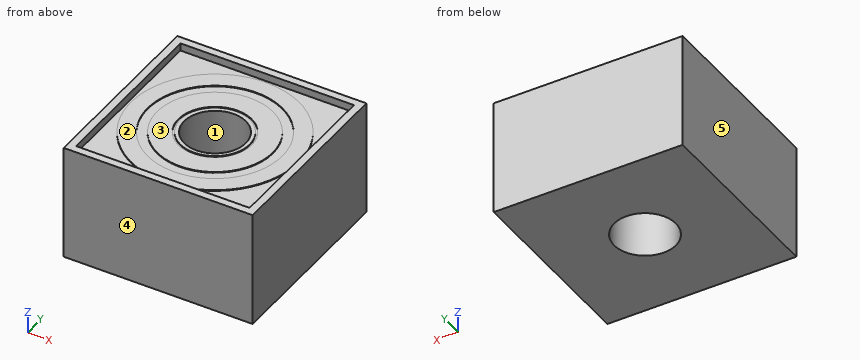
```python
from build123d import *

# Parameters (mm, degrees)
SKETCH2_W                = 24.5
SKETCH2_H                = 24.5
SKETCH2_W_2              = 22.5
SKETCH2_H_2              = 22.5
BOSS_EXTRUDE1_DEPTH      = 15
SKETCH3_W                = 22.5
SKETCH3_H                = 22.5
BOSS_EXTRUDE2_DEPTH      = 14
BOSS_EXTRUDE4_DEPTH      = 0.1
BOSS_EXTRUDE4_DEPTH_BACK = 6.9
SKETCH4_R                = 10.9
SKETCH4_R_2              = 8.730342775
SKETCH4_R_3              = 7.5
SKETCH4_R_4              = 4.75
SKETCH4_R_5              = 4.5
SKETCH4_R_6              = 4
CUT_EXTRUDE1_START       = -15
SKETCH6_R                = 4
CUT_EXTRUDE1_DEPTH       = 15


with BuildPart() as part:
    # Sketch2 → Boss-Extrude1 (new body)
    with BuildSketch(Plane.XY):
        Rectangle(SKETCH2_W, SKETCH2_H)
        Rectangle(SKETCH2_W_2, SKETCH2_H_2, mode=Mode.SUBTRACT)
    extrude(amount=BOSS_EXTRUDE1_DEPTH)

    # Sketch3 → Boss-Extrude2 (add)
    with BuildSketch(Plane.XY):
        Rectangle(SKETCH3_W, SKETCH3_H)
    extrude(amount=BOSS_EXTRUDE2_DEPTH)

    # Sketch4 → Boss-Extrude4 (add, two sides: drawn at the far end of the back side and taken through both)
    # profile 1 of 3: a face of its own
    with BuildSketch(Plane.XY.offset(14).offset(-BOSS_EXTRUDE4_DEPTH_BACK)):
        Circle(SKETCH4_R)
        Circle(SKETCH4_R_2, mode=Mode.SUBTRACT)
    # profile 2 of 3: a face of its own
    with BuildSketch(Plane.XY.offset(14).offset(-BOSS_EXTRUDE4_DEPTH_BACK)):
        Circle(SKETCH4_R_3)
        Circle(SKETCH4_R_4, mode=Mode.SUBTRACT)
    # profile 3 of 3: a face of its own
    with BuildSketch(Plane.XY.offset(14).offset(-BOSS_EXTRUDE4_DEPTH_BACK)):
        Circle(SKETCH4_R_5)
        Circle(SKETCH4_R_6, mode=Mode.SUBTRACT)
    extrude(amount=BOSS_EXTRUDE4_DEPTH + BOSS_EXTRUDE4_DEPTH_BACK)

    # Sketch6 → Cut-Extrude1 (cut)
    with BuildSketch(Plane.XY.offset(14).offset(CUT_EXTRUDE1_START)):
        Circle(SKETCH6_R)
    extrude(amount=CUT_EXTRUDE1_DEPTH, mode=Mode.SUBTRACT)


solid = part.part
```
Geometry check sheet. Reference: the model listing, model coordinates, mm. Face numbers are marked on the shaded views. A direction names the side the tool comes from. Give positions to 0.01 mm unless a question says otherwise; leave off trailing zeros. Write each loop counter-clockwise with the first axis right and the second up, starting at its lowest first coordinate (ties: lowest second). Pieces come first, ordered by that corner, then holes. Notation, with made-up numbers: (-20.5, -9.5) -> (31.5, -9.5) arc R34 ccw to (31.5, 26.5) -> close; hole circle Ø3 at (33.25, -29). An arc over 180 degrees is marked (long way). Use one line per item in the form item = value.
Item 1: Access from +Z, -Z, +X, -X, +Y, -Y to the whole of each face (thin tool, end or side, straight path). Record for the marked faces 1 and 2.
Results list:
face_1 = +Z, -Z
face_2 = +Z
Item 2: Sectioned sample at C-C on z = 13.25. Enter the section's corners in (x, y).
Results list:
outline = (-12.25, -12.25) -> (12.25, -12.25) -> (12.25, 12.25) -> (-12.25, 12.25) -> close; hole circle Ø8 at (0, 0)
Item 3: Mould release check, pull along X, two halves, no side actions. Record for the marked faces 3, 4 and 5: released by +X, released by -X, zero draft, split by the parting line, or undercut.
Results list:
face_3 = undercut
face_4 = zero draft
face_5 = released by -X
Item 4: Depth check by flat-ended pin: pin 1 Ø12 at (x, y) = (8.5, -6.5) entering from -Z; pin 2 Ø4.5 at (x, y) = (-2.5, 2) entering from +Z. Enter the tip coordinate at first touch or a pass-through.
Results list:
pin_1 = 0
pin_2 = 14.1
Item 5: Scan lines: line 1 (Y direction, x = 0, z = 5.75); line 2 (X direction, y = -1.75, z = 6.25). Record each from-to range of solid material in increasing order.
Results list:
line_1 = -12.25 to -4, 4 to 12.25
line_2 = -12.25 to -3.6, 3.6 to 12.25
Item 6: Sectioned sample at D-D on y = 10. Enter the section's corners in (x, z), plus the area to 3 significant figures.
Results list:
outline = (-12.25, 0) -> (12.25, 0) -> (12.25, 15) -> (11.25, 15) -> (11.25, 14) -> (4.34, 14) -> (4.34, 14.1) -> (-4.34, 14.1) -> (-4.34, 14) -> (-11.25, 14) -> (-11.25, 15) -> (-12.25, 15) -> close
area = 346 mm2
